Check sheet for the modelled part. Datum: model origin and axes. Units: mm. Coordinates: 2 decimals unless noted, no trailing zeros. Loops run counter-clockwise (first coordinate to the right, second up) from the corner with the lowest first, then second, coordinate; pieces in that order, holes last. Notation, with made-up numbers: M 31,31 L 43,31 A11 cw 43,52 Z; hole C 84,-12.75 d8. An arc over 180 degrees is marked long. Return JSON: item names as keys, results as strings.
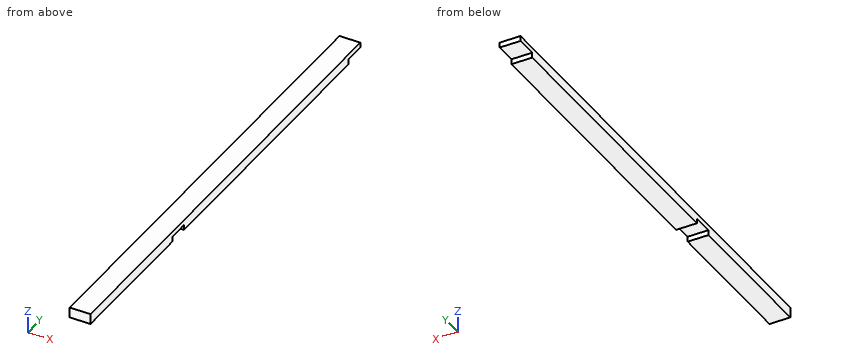
Autodesk Inventor part; units mm, degrees
ref_plane "YZ Plane" through (0, 0, 0) normal (1, 0, 0) x (0, 1, 0)
ref_plane "XZ Plane" through (0, 0, 0) normal (0, 1, 0) x (-1, 0, 0)
ref_plane "XY Plane" through (0, 0, 0) normal (0, 0, 1) x (1, 0, 0)
sketch "Sketch1" plane through (0, 0, 0) normal (0, 0, 1) x (1, 0, 0)
  line L0 (657.7721, 961.825) -> (695.8721, 961.825)
  line L1 (695.8721, 961.825) -> (695.8721, 82.35)
  line L2 (695.8721, 82.35) -> (657.7721, 82.35)
  line L3 (657.7721, 82.35) -> (657.7721, 961.825)
  point P0 (0, 0)
  dimension "d0" = 879.475
  dimension "d1" = 38.1
extrude "Board" add sketch "Sketch1" along normal blind 19.05
sketch "Sketch2" plane through (0, 0, 0) normal (0, 0, -1) x (-1, 0, 0)
  line L0 (-695.8721, 82.35) -> (-695.8721, 961.825)
  line L1 (-657.7721, 961.825) -> (-657.7721, 82.35)
  line L2 (-695.8721, 961.825) -> (-657.7721, 961.825)
  line L3 (-657.7721, 961.825) -> (-657.7721, 923.725)
  line L4 (-657.7721, 923.725) -> (-695.8721, 923.725)
  line L5 (-695.8721, 923.725) -> (-695.8721, 961.825)
  point P0 (0, 0)
  dimension "d4" = 38.1
extrude "Top Notch" cut sketch "Sketch2" against normal blind 9.525
sketch "Sketch3" plane through (0, 0, 0) normal (0, 0, -1) x (-1, 0, 0)
  line L0 (-695.8721, 923.725) -> (-695.8721, 82.35)
  line L1 (-657.7721, 961.825) -> (-657.7721, 82.35)
  line L2 (-695.8721, 387.15) -> (-657.7721, 387.15)
  line L3 (-657.7721, 387.15) -> (-657.7721, 349.05)
  line L4 (-657.7721, 349.05) -> (-695.8721, 349.05)
  line L5 (-695.8721, 349.05) -> (-695.8721, 387.15)
  line L6 (-695.8721, 82.35) -> (-657.7721, 82.35)
  line L7 (-695.8721, 961.825) -> (-657.7721, 961.825)
  point P0 (0, 0)
  dimension "d7" = 38.1
  dimension "d11" = 574.675
extrude "Bottom Notch" cut sketch "Sketch3" against normal blind 9.525 contours L2 L1 L4 L0
properties part number "Cabinet Support Frame Center Vertical Bar"
1) Section check B-B on x = 684.5. Record the cut outline in (y, z) (3 decimals), then the cut area to 3 significant figures.
Answers:
{"outline": "M 82.35,0 L 349.05,0 L 349.05,9.525 L 387.15,9.525 L 387.15,0 L 923.725,0 L 923.725,9.525 L 961.825,9.525 L 961.825,19.05 L 82.35,19.05 Z", "area": "16,000 mm²"}
2) Go/stop test with flat-tipped pins: pin 1 Ø1 at (x, z) = (678.5, 8.5) entering from +Y (3 decimals); pin 2 Ø19 at (x, y) = (675, 365) entering from -Z (3 decimals). Record where each tip stops, or that it passes through.
Answers:
{"pin 1": "y = 923.725", "pin 2": "z = 9.525"}
3) Section check A-A on z = 4.75. Record the cut outline in (x, y) (3 decimals), then the cut area to 3 significant figures.
Answers:
{"outline": "M 657.772,82.35 L 695.872,82.35 L 695.872,349.05 L 657.772,349.05 Z; M 657.772,387.15 L 695.872,387.15 L 695.872,923.725 L 657.772,923.725 Z", "area": "30,600 mm²"}
4) Scan lines: line 1 along Y through (x, z) = (666.5, 2) (3 decimals); line 2 along Z through (x, y) = (688, 359) (3 decimals). Record each from-to range of solid material in increasing order. Write a range as [from, to].
Answers:
{"line 1": "[82.35, 349.05], [387.15, 923.725]", "line 2": "[9.525, 19.05]"}
